Check sheet for the modelled part. Datum: model origin and axes. Units: mm. A direction names the side the tool comes from. Give positions to 0.01 mm unless a question says otherwise; leave off trailing zeros. Order: outer loops, then holes, each group sorted by start corner. A loop starts at its lowest first (then second) coordinate and runs counter-clockwise, first axis right, second up. Notation, with made-up numbers: (25.25, -27.75) -> (40.25, -27.75) arc R11 ccw to (40.25, -20.75) -> close; hole circle Ø10 at (47, 59.25). An arc over 180 degrees is marked (long way). Answer in a Markdown table with one row per item. Add a question column.
(1) Cross-section at A-A (x = -8). Record the cut outline in (y, z) (3 decimals), then the cut area to 3 significant figures.
(2) Set-up check for faces 1 (the face through (13.675, -0.011, 1.479)), 2 (the face through (61.049, 0, 1)): record each of +Z, -Z, +X, -X, +Y, -Y from which the full face is reachable in a straight line by a thin tool's end or side.
(3) Go/stop test with a flat-tipped pin: pin 1 (6 mm diameter, centred on x = 37, y = 5, fed in from -Z). Record where the tip stops, or that it passes through.
(4) Release check for a two-part mould opening along Y. For faces 3 (the face through (23, 2, 3)), 4 (the face through (26.325, 0.011, 1.479)) record: released by +Y, released by -Y, zero draft, split by the parting line, or undercut.
(5) Cross-section at B-B (y = 0). State how many separate pieces and enclosed holes the cut face has, then the cut area to 3 significant figures.
(6) Thickness scan on L1, parallel to Y at x = -8, z = 0.95 (3 decimals); L2, parallel to Y at x = 42, z = 2.15. Record the ranges inside material, lowest first. Write a range as [from, to].
```python
from build123d import *

# Parameters (mm, degrees)
F0_W     = 75.035495
F0_H     = 15.439995
F0_R     = 2.325
F1_DEPTH = 3


with BuildPart() as f1:
    # F0 (on Top) → F1 (new body)
    with BuildSketch(Plane.XY):
        with Locations((23.531661, -0.09854)):
            Rectangle(F0_W, F0_H)
        with Locations((-8, 0)):
            Circle(F0_R, mode=Mode.SUBTRACT)
        with BuildLine():
            Line((0.8, 2.183031), (0.8, 1.1))
            ThreePointArc((0.8, 1.1), (0.887868, 0.887868), (1.1, 0.8))
            Line((1.1, 0.8), (2.183031, 0.8))
            ThreePointArc((2.183031, 0.8), (2.325, 0), (2.183031, -0.8))
            Line((2.183031, -0.8), (1.1, -0.8))
            ThreePointArc((1.1, -0.8), (0.887868, -0.887868), (0.8, -1.1))
            Line((0.8, -1.1), (0.8, -2.183031))
            ThreePointArc((0.8, -2.183031), (0, -2.325), (-0.8, -2.183031))
            Line((-0.8, -2.183031), (-0.8, -1.1))
            ThreePointArc((-0.8, -1.1), (-0.887868, -0.887868), (-1.1, -0.8))
            Line((-1.1, -0.8), (-2.183031, -0.8))
            ThreePointArc((-2.183031, -0.8), (-2.325, 0), (-2.183031, 0.8))
            Line((-2.183031, 0.8), (-1.1, 0.8))
            ThreePointArc((-1.1, 0.8), (-0.887868, 0.887868), (-0.8, 1.1))
            Line((-0.8, 1.1), (-0.8, 2.183031))
            ThreePointArc((-0.8, 2.183031), (0, 2.325), (0.8, 2.183031))
        make_face(mode=Mode.SUBTRACT)
        with BuildLine():
            ThreePointArc((8.8, -2.183031), (8, -2.325), (7.2, -2.183031))
            Line((7.2, -2.183031), (7.2, -1.1))
            ThreePointArc((7.2, -1.1), (7.112132, -0.887868), (6.9, -0.8))
            Line((6.9, -0.8), (5.816969, -0.8))
            ThreePointArc((5.816969, -0.8), (5.675, 0), (5.816969, 0.8))
            Line((5.816969, 0.8), (6.9, 0.8))
            ThreePointArc((6.9, 0.8), (7.112132, 0.887868), (7.2, 1.1))
            Line((7.2, 1.1), (7.2, 2.183031))
            ThreePointArc((7.2, 2.183031), (8, 2.325), (8.8, 2.183031))
            Line((8.8, 2.183031), (8.8, 1.1))
            ThreePointArc((8.8, 1.1), (8.887868, 0.887868), (9.1, 0.8))
            Line((9.1, 0.8), (10.183031, 0.8))
            ThreePointArc((10.183031, 0.8), (10.325, 0), (10.183031, -0.8))
            Line((10.183031, -0.8), (9.1, -0.8))
            ThreePointArc((9.1, -0.8), (8.887868, -0.887868), (8.8, -1.1))
            Line((8.8, -1.1), (8.8, -2.183031))
        make_face(mode=Mode.SUBTRACT)
        with BuildLine():
            ThreePointArc((16.8, -2.183031), (16, -2.325), (15.2, -2.183031))
            Line((15.2, -2.183031), (15.2, -1.1))
            ThreePointArc((15.2, -1.1), (15.112132, -0.887868), (14.9, -0.8))
            Line((14.9, -0.8), (13.816969, -0.8))
            ThreePointArc((13.816969, -0.8), (13.675, 0), (13.816969, 0.8))
            Line((13.816969, 0.8), (14.9, 0.8))
            ThreePointArc((14.9, 0.8), (15.112132, 0.887868), (15.2, 1.1))
            Line((15.2, 1.1), (15.2, 2.183031))
            ThreePointArc((15.2, 2.183031), (16, 2.325), (16.8, 2.183031))
            Line((16.8, 2.183031), (16.8, 1.1))
            ThreePointArc((16.8, 1.1), (16.887868, 0.887868), (17.1, 0.8))
            Line((17.1, 0.8), (18.183031, 0.8))
            ThreePointArc((18.183031, 0.8), (18.325, 0), (18.183031, -0.8))
            Line((18.183031, -0.8), (17.1, -0.8))
            ThreePointArc((17.1, -0.8), (16.887868, -0.887868), (16.8, -1.1))
            Line((16.8, -1.1), (16.8, -2.183031))
        make_face(mode=Mode.SUBTRACT)
        with BuildLine():
            ThreePointArc((24.8, -2.183031), (24, -2.325), (23.2, -2.183031))
            Line((23.2, -2.183031), (23.2, -1.1))
            ThreePointArc((23.2, -1.1), (23.112132, -0.887868), (22.9, -0.8))
            Line((22.9, -0.8), (21.816969, -0.8))
            ThreePointArc((21.816969, -0.8), (21.675, 0), (21.816969, 0.8))
            Line((21.816969, 0.8), (22.9, 0.8))
            ThreePointArc((22.9, 0.8), (23.112132, 0.887868), (23.2, 1.1))
            Line((23.2, 1.1), (23.2, 2.183031))
            ThreePointArc((23.2, 2.183031), (24, 2.325), (24.8, 2.183031))
            Line((24.8, 2.183031), (24.8, 1.1))
            ThreePointArc((24.8, 1.1), (24.887868, 0.887868), (25.1, 0.8))
            Line((25.1, 0.8), (26.183031, 0.8))
            ThreePointArc((26.183031, 0.8), (26.325, 0), (26.183031, -0.8))
            Line((26.183031, -0.8), (25.1, -0.8))
            ThreePointArc((25.1, -0.8), (24.887868, -0.887868), (24.8, -1.1))
            Line((24.8, -1.1), (24.8, -2.183031))
        make_face(mode=Mode.SUBTRACT)
        with BuildLine():
            ThreePointArc((32.8, -2.183031), (32, -2.325), (31.2, -2.183031))
            Line((31.2, -2.183031), (31.2, -1.1))
            ThreePointArc((31.2, -1.1), (31.112132, -0.887868), (30.9, -0.8))
            Line((30.9, -0.8), (29.816969, -0.8))
            ThreePointArc((29.816969, -0.8), (29.675, 0), (29.816969, 0.8))
            Line((29.816969, 0.8), (30.9, 0.8))
            ThreePointArc((30.9, 0.8), (31.112132, 0.887868), (31.2, 1.1))
            Line((31.2, 1.1), (31.2, 2.183031))
            ThreePointArc((31.2, 2.183031), (32, 2.325), (32.8, 2.183031))
            Line((32.8, 2.183031), (32.8, 1.1))
            ThreePointArc((32.8, 1.1), (32.887868, 0.887868), (33.1, 0.8))
            Line((33.1, 0.8), (34.183031, 0.8))
            ThreePointArc((34.183031, 0.8), (34.325, 0), (34.183031, -0.8))
            Line((34.183031, -0.8), (33.1, -0.8))
            ThreePointArc((33.1, -0.8), (32.887868, -0.887868), (32.8, -1.1))
            Line((32.8, -1.1), (32.8, -2.183031))
        make_face(mode=Mode.SUBTRACT)
        with BuildLine():
            ThreePointArc((40.8, -2.183031), (40, -2.325), (39.2, -2.183031))
            Line((39.2, -2.183031), (39.2, -1.1))
            ThreePointArc((39.2, -1.1), (39.112132, -0.887868), (38.9, -0.8))
            Line((38.9, -0.8), (37.816969, -0.8))
            ThreePointArc((37.816969, -0.8), (37.675, 0), (37.816969, 0.8))
            Line((37.816969, 0.8), (38.9, 0.8))
            ThreePointArc((38.9, 0.8), (39.112132, 0.887868), (39.2, 1.1))
            Line((39.2, 1.1), (39.2, 2.183031))
            ThreePointArc((39.2, 2.183031), (40, 2.325), (40.8, 2.183031))
            Line((40.8, 2.183031), (40.8, 1.1))
            ThreePointArc((40.8, 1.1), (40.887868, 0.887868), (41.1, 0.8))
            Line((41.1, 0.8), (42.183031, 0.8))
            ThreePointArc((42.183031, 0.8), (42.325, 0), (42.183031, -0.8))
            Line((42.183031, -0.8), (41.1, -0.8))
            ThreePointArc((41.1, -0.8), (40.887868, -0.887868), (40.8, -1.1))
            Line((40.8, -1.1), (40.8, -2.183031))
        make_face(mode=Mode.SUBTRACT)
        with BuildLine():
            ThreePointArc((48.8, -2.183031), (48, -2.325), (47.2, -2.183031))
            Line((47.2, -2.183031), (47.2, -1.1))
            ThreePointArc((47.2, -1.1), (47.112132, -0.887868), (46.9, -0.8))
            Line((46.9, -0.8), (45.816969, -0.8))
            ThreePointArc((45.816969, -0.8), (45.675, 0), (45.816969, 0.8))
            Line((45.816969, 0.8), (46.9, 0.8))
            ThreePointArc((46.9, 0.8), (47.112132, 0.887868), (47.2, 1.1))
            Line((47.2, 1.1), (47.2, 2.183031))
            ThreePointArc((47.2, 2.183031), (48, 2.325), (48.8, 2.183031))
            Line((48.8, 2.183031), (48.8, 1.1))
            ThreePointArc((48.8, 1.1), (48.887868, 0.887868), (49.1, 0.8))
            Line((49.1, 0.8), (50.183031, 0.8))
            ThreePointArc((50.183031, 0.8), (50.325, 0), (50.183031, -0.8))
            Line((50.183031, -0.8), (49.1, -0.8))
            ThreePointArc((49.1, -0.8), (48.887868, -0.887868), (48.8, -1.1))
            Line((48.8, -1.1), (48.8, -2.183031))
        make_face(mode=Mode.SUBTRACT)
        with BuildLine():
            ThreePointArc((56.8, -2.183031), (56, -2.325), (55.2, -2.183031))
            Line((55.2, -2.183031), (55.2, -1.1))
            ThreePointArc((55.2, -1.1), (55.112132, -0.887868), (54.9, -0.8))
            Line((54.9, -0.8), (53.816969, -0.8))
            ThreePointArc((53.816969, -0.8), (53.675, 0), (53.816969, 0.8))
            Line((53.816969, 0.8), (54.9, 0.8))
            ThreePointArc((54.9, 0.8), (55.112132, 0.887868), (55.2, 1.1))
            Line((55.2, 1.1), (55.2, 2.183031))
            ThreePointArc((55.2, 2.183031), (56, 2.325), (56.8, 2.183031))
            Line((56.8, 2.183031), (56.8, 1.1))
            ThreePointArc((56.8, 1.1), (56.887868, 0.887868), (57.1, 0.8))
            Line((57.1, 0.8), (58.183031, 0.8))
            ThreePointArc((58.183031, 0.8), (58.325, 0), (58.183031, -0.8))
            Line((58.183031, -0.8), (57.1, -0.8))
            ThreePointArc((57.1, -0.8), (56.887868, -0.887868), (56.8, -1.1))
            Line((56.8, -1.1), (56.8, -2.183031))
        make_face(mode=Mode.SUBTRACT)
    extrude(amount=F1_DEPTH)


solid = f1.part
```
Answer below:
| question | item | result |
|---|---|---|
| 1 | outline | (-7.819, 0) -> (-2.325, 0) -> (-2.325, 3) -> (-7.819, 3) -> close; (2.325, 0) -> (7.621, 0) -> (7.621, 3) -> (2.325, 3) -> close |
| 1 | area | 32.4 mm² |
| 2 | face 1 | +Z, -Z |
| 2 | face 2 | +Z, -Z, +X, +Y, -Y |
| 3 | pin 1 | stops at z = 0 |
| 4 | face 3 | zero draft |
| 4 | face 4 | undercut |
| 5 | separate pieces | 10 |
| 5 | enclosed holes | 0 |
| 5 | area | 99.6 mm² |
| 6 | L1 | y = [-7.819, -2.325], [2.325, 7.621] |
| 6 | L2 | y = [-7.82, -0.8], [0.8, 7.62] |
